Source: CAD feature listing. Evaluate the final solid. Frame: model axes, mm. Face numbers are marked on the shaded views. A direction names the side the tool comes from. Give positions to 0.01 mm unless a question says otherwise; leave off trailing zeros. Order: outer loops, then holes, each group sorted by start corner. A loop starts at its lowest first (then second) coordinate and runs counter-clockwise, first axis right, second up.
1) Access query for the marked faces 4, 5 and 6. Directions: +Z, -Z, +X, -X, +Y, -Y. A direction counts if a zero-diameter tool reaches every point of the face in a straight line with its end or side. Return the directions, or none.
2) First-contact query: P1, Ø1, axis at x = -1, z = -1.5, coming from the +Y side; P2, Ø0.6, axis at y = -0.5, z = 2.5, coming from the +X side. Flat tips, straight axial feed; report the tip coordinate or a pass-through.
3) Section A-A, the plane z = 2.25. Return loops of the section in (x, y).
4) Section B-B, the plane y = 0. Return loops of the section in (x, z).
5) Section D-D, the plane z = 0.25. Return loops of the section in (x, y).
6) Section C-C, the plane x = 1.1. Return loops of the section in (y, z).
7) Material intervals for line 1 (Y direction, x = 2.45, z = 0.5); line 2 (Z direction, x = -1.1, y = -1.9); line 3 (X direction, y = 0.5, z = 2), sorted ascending.
8) Draft query along X for the marked faces 1, 2 and 3. Return one class per face: released by +X, released by -X, zero draft, split by the parting line, or undercut.
Autodesk Inventor part; units mm, degrees
ref_plane "YZ Plane" through (0, 0, 0) normal (1, 0, 0) x (0, 1, 0)
ref_plane "XZ Plane" through (0, 0, 0) normal (0, 1, 0) x (-1, 0, 0)
ref_plane "XY Plane" through (0, 0, 0) normal (0, 0, 1) x (1, 0, 0)
sketch "スケッチ1" plane through (0, 0, 0) normal (0, 0, 1) x (1, 0, 0)
  circle A0 centre (0, 0) radius 1.5
  dimension "d0" = 3
extrude "押し出し1" add sketch "スケッチ1" against normal blind 5
sketch "スケッチ2" plane through (0, 0, 0) normal (0, 0, 1) x (1, 0, 0)
  circle A0 centre (0, 0) radius 2.75
  dimension "d3" = 5.5
extrude "押し出し2" add sketch "スケッチ2" along normal blind 3
sketch "スケッチ3" plane through (0, 0, 3) normal (0, 0, 1) x (1, 0, 0)
  line L0 (0, 1.4434) -> (1.25, 0.7217)
  line L1 (1.25, 0.7217) -> (1.25, -0.7217)
  line L2 (1.25, -0.7217) -> (0, -1.4434)
  line L3 (0, -1.4434) -> (-1.25, -0.7217)
  line L4 (-1.25, -0.7217) -> (-1.25, 0.7217)
  line L5 (-1.25, 0.7217) -> (0, 1.4434)
  point P0 (0, 0)
  point P1 (0, 0)
  dimension "d6" = 2.5
extrude "押し出し3" cut sketch "スケッチ3" against normal blind 1.3
thread "ねじ1"
properties part number "M3キャップボルト5" material "鋼、高強度、低合金"
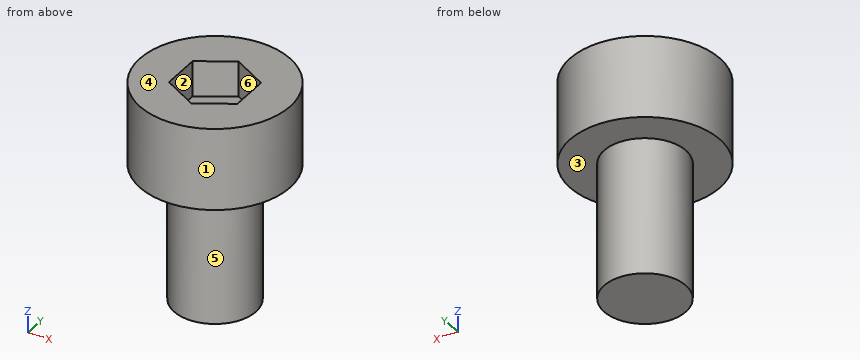
From the geometry:
1. face 4: +Z, +X, -X, +Y, -Y
1. face 5: -Z
1. face 6: +Z
2. P1: stops at y = 1.41
2. P2: stops at x = 2.74
3. outline: circle Ø5.5 at (0, 0); hole (-1.25, -0.72) - (0, -1.44) - (1.25, -0.72) - (1.25, 0.72) - (0, 1.44) - (-1.25, 0.72) - close
4. outline: (-2.75, 0) - (-1.5, 0) - (-1.5, -5) - (1.5, -5) - (1.5, 0) - (2.75, 0) - (2.75, 3) - (1.25, 3) - (1.25, 1.7) - (-1.25, 1.7) - (-1.25, 3) - (-2.75, 3) - close
5. outline: circle Ø5.5 at (0, 0)
6. outline: (-2.52, 0) - (-1.02, 0) - (-1.02, -5) - (1.02, -5) - (1.02, 0) - (2.52, 0) - (2.52, 3) - (0.81, 3) - (0.81, 1.7) - (-0.81, 1.7) - (-0.81, 3) - (-2.52, 3) - close
7. line 1: y = -1.25 to 1.25
7. line 2: z = 0 to 3
7. line 3: x = -2.7 to -1.25, 1.25 to 2.7
8. face 1: split by the parting line
8. face 2: undercut
8. face 3: zero draft
